Autodesk Inventor part; units mm, degrees
ref_plane "YZ Plane" through (0, 0, 0) normal (1, 0, 0) x (0, 1, 0)
ref_plane "XZ Plane" through (0, 0, 0) normal (0, 1, 0) x (-1, 0, 0)
ref_plane "XY Plane" through (0, 0, 0) normal (0, 0, 1) x (1, 0, 0)
sketch "Sketch1" plane through (0, 0, 0) normal (0, 0, 1) x (1, 0, 0)
  line L0 (-12.1708, 16.0073) -> (13.2292, 16.0073)
  line L1 (13.2292, 16.0073) -> (13.2292, -34.7927)
  line L2 (13.2292, -34.7927) -> (-12.1708, -34.7927)
  line L3 (-12.1708, -34.7927) -> (-12.1708, 16.0073)
  line L4 (11.9592, 14.7373) -> (-10.9008, 14.7373)
  line L5 (-10.9008, 14.7373) -> (-10.9008, -33.5227)
  line L6 (-10.9008, -33.5227) -> (11.9592, -33.5227)
  line L7 (11.9592, -33.5227) -> (11.9592, 14.7373)
  point P0 (0, 0)
  dimension "d0" = 25.4
  dimension "d1" = 50.8
  dimension "d2" = 1.27
extrude "Extrusion1" add sketch "Sketch1" along normal blind 508
sketch "Sketch2" plane through (-12.1708, 16.0073, 0) normal (0, 1, 0) x (1, 0, 0)
  circle A0 centre (12.7, -12.7) radius 1.7272
  line L0 (25.4, 0) -> (0, 0)
  line L1 (0, 0) -> (0, -508)
  point P0 (12.1708, 0)
  dimension "d5" = 3.4544
  dimension "d6" = 12.7
  dimension "d7" = 12.7
extrude "Extrusion2" cut sketch "Sketch2" against normal through all
pattern_linear "Rectangular Pattern1" count 20 spacing 25.4 along (0, 0, 1) of "Extrusion2"
equation "\"d3\" = d13"
equation "\"d13\" = 508"
properties part number "VerseFrame 20in"
Build history of the part. All positions in model axes, mm. A direction names the side the tool comes from. Give positions to 0.01 mm unless a question says otherwise; leave off trailing zeros. Order: outer loops, then holes, each group sorted by start corner. A loop starts at its lowest first (then second) coordinate and runs counter-clockwise, first axis right, second up. Notation, with made-up numbers: M 44,-7.5 L 59,-7.5 A20 cw 59,13.5 Z; hole C -6,-5.5 d5. An arc over 180 degrees is marked long. Use one line per item in the form item = value.
1) Tool access for faces 5 (the face through (-12, -9, 0)), 6 (the face through (1, 14.737, 250)): list every direction of +Z, -Z, +X, -X, +Y, -Y with a clear straight run to the whole face (end or side of a thin tool).
Calculated:
face_5 = -Z, +X, -X, +Y, -Y
face_6 = +Z, -Z
2) Probe probe 1 along X at (y, z) = (15, 165); probe 2 along X at (y, z) = (14, 450.5); probe 3 along Y at (x, z) = (6, 78). List the from-to ranges inside material, lowest first.
Calculated:
probe_1 = -12.17 to -1.2, 2.25 to 13.23
probe_2 = -12.17 to -10.9, 11.96 to 13.23
probe_3 = -34.79 to -33.52, 14.74 to 16.01
3) Saw through at A-A (y = -15.5). Give the cut face in (x, z).
Calculated:
outline = M -12.17,0 L -10.9,0 L -10.9,508 L -12.17,508 Z; M 11.96,0 L 13.23,0 L 13.23,508 L 11.96,508 Z
4) Saw through at B-B (x = 7.25). Give the cut face in (y, z), plus the area to 3 significant figures.
Calculated:
outline = M -34.79,0 L -33.52,0 L -33.52,508 L -34.79,508 Z; M 14.74,0 L 16.01,0 L 16.01,508 L 14.74,508 Z
area = 1,290 mm2
5) Drop a flat-ended pin along its axis: pin 1 (4 mm diameter, centred on x = 0.53, z = 317.5, fed in from +Y). Give the stop position or say it passes through.
Calculated:
pin_1 = 16.01
6) Saw through at C-C (z = 122.5). Give the cut face in (x, y).
Calculated:
outline = M -12.17,-34.79 L 13.23,-34.79 L 13.23,16.01 L -12.17,16.01 Z; hole M -10.9,-33.52 L 11.96,-33.52 L 11.96,14.74 L -10.9,14.74 Z
7) Two-plate mould, pull along Y, no slides. Class faces 1 (the face through (0, 16.007, 250)), 2 (the face through (-10.901, -9, 250)), 3 (the face through (0, -33.523, 250)), 4 (the face through (13.229, -9, 250)): released by +Y, released by -Y, zero draft, split by the parting line, or undercut.
Calculated:
face_1 = released by +Y
face_2 = undercut
face_3 = undercut
face_4 = zero draft
